from build123d import *

# Parameters (mm, degrees)
F3_W          = 55
F3_H          = 55
F4_DEPTH      = 6
F7_W          = 12.7
F7_H          = 6
F8_DEPTH      = 6
F10_W         = 12.7
F10_H         = 6
F11_DEPTH     = 6
F13_W         = 12.7
F13_H         = 6
F14_DEPTH     = 6
F16_W         = 12.7
F16_H         = 6
F17_DEPTH     = 6
F19_D         = 5
F21_D         = 5
F23_D         = 5
F25_D         = 5
F26_T4_DEPTH  = 133
F26_T10_DEPTH = 133
F26_T15_DEPTH = 133
F26_T21_DEPTH = 133
F26_T27_DEPTH = 133
F26_T33_DEPTH = 133
F26_T38_DEPTH = 133
F26_T44_DEPTH = 133
F26_T49_DEPTH = 133
F26_T55_DEPTH = 133
F26_T61_DEPTH = 133
F26_T66_DEPTH = 133
F27_R         = 6.34999


# Not quite as in the source:
# - a fillet or chamfer that OpenCascade refuses, or shapes differently, is made with other operations: its cross-section is extruded or revolved along the edge and cut away or added
# - a fillet or chamfer is up to 0.001 mm smaller than in the source, because OpenCascade refuses the exact size


with BuildPart() as f1:
    # F0 (on Front) → F1 (revolve)
    with BuildSketch(Plane.XZ):
        with BuildLine():
            Line((0, 0), (0, -32.5))
            add(Edge.make_bspline(
                [(0, -32.5), (25, -32.5), (25, 0)],
                knots=[0, 0, 0, 1.5707963268, 1.5707963268, 1.5707963268], degree=2, weights=[1, 0.7071067812, 1]))
            Line((25, 0), (0, 0))
        make_face()
        with BuildLine():
            Line((0, 0), (25, 0))
            add(Edge.make_bspline(
                [(25, 0), (25, 32.5), (0, 32.5)],
                knots=[1.5707963268, 1.5707963268, 1.5707963268, 3.1415926536, 3.1415926536, 3.1415926536], degree=2, weights=[1, 0.7071067812, 1]))
            Line((0, 32.5), (0, 0))
        make_face()
    revolve(axis=Axis((0, 0, 0), (0, 0, -1)))


with BuildPart() as f4:
    # F3 (on offset) → F4 (new body)
    with BuildSketch(Plane.XY.offset(19.05)):
        Rectangle(F3_W, F3_H)
    extrude(amount=-F4_DEPTH)

    # F5: cut F1
    add(f1.part, mode=Mode.SUBTRACT)

    # F7 (on offset) → F8 (join)
    with BuildSketch(Plane.XZ.offset(27.5)):
        with Locations((0, 16.0963926464)):
            Rectangle(F7_W, F7_H)
    extrude(amount=F8_DEPTH)

    # F10 (on offset) → F11 (join)
    with BuildSketch(Plane.YZ.offset(27.5)):
        with Locations((0, 16.087366268)):
            Rectangle(F10_W, F10_H)
    extrude(amount=F11_DEPTH)

    # F13 (on offset) → F14 (join)
    with BuildSketch(Plane.XZ.offset(-27.5)):
        with Locations((0, 16.07888937)):
            Rectangle(F13_W, F13_H)
    extrude(amount=-F14_DEPTH)

    # F16 (on offset) → F17 (join)
    with BuildSketch(Plane.YZ.offset(-27.5)):
        with Locations((0, 16.0636380315)):
            Rectangle(F16_W, F16_H)
    extrude(amount=-F17_DEPTH)

    # F19 (through all)
    with Locations(Plane.XY.offset(19.07888937)):
        with Locations((0, 28.8921689615)):
            Hole(F19_D / 2)

    # F21 (through all)
    with Locations(Plane.XY.offset(19.0636380315)):
        with Locations((-28.8809893653, 0)):
            Hole(F21_D / 2)

    # F23 (through all)
    with Locations(Plane.XY.offset(19.087366268)):
        with Locations((28.8808012381, 0)):
            Hole(F23_D / 2)

    # F25 (through all)
    with Locations(Plane.XY.offset(19.0963926464)):
        with Locations((0, -28.8607433438)):
            Hole(F25_D / 2)

    # F26: fillet of radius 25.4 on 4 edges, made by hand


with BuildPart() as f26_tool2:
    # F26_s3 → F26_t4 (new body)
    with BuildSketch(Plane.XY.offset(82.55)):
        with BuildLine():
            ThreePointArc((-27.5, 2.1), (-20.0605122421, 20.0605122421), (-2.1, 27.5))
            Line((-2.1, 27.5), (-27.5, 27.5))
            Line((-27.5, 27.5), (-27.5, 2.1))
        make_face()
    extrude(amount=-F26_T4_DEPTH)

    split(bisect_by=Plane.XZ.offset(-6.35), keep=Keep.BOTTOM)

    split(bisect_by=Plane.YZ.offset(-6.35), keep=Keep.BOTTOM)


with BuildPart() as f4_1:
    add(f4.part)

    # F26_t1: cut F26_tool2
    add(f26_tool2.part, mode=Mode.SUBTRACT)


with BuildPart() as f26_tool8:
    # F26_s9 → F26_t10 (new body)
    with BuildSketch(Plane.XY.offset(82.55)):
        with BuildLine():
            ThreePointArc((-27.5, 2.1), (-20.0605122421, 20.0605122421), (-2.1, 27.5))
            Line((-2.1, 27.5), (-27.5, 27.5))
            Line((-27.5, 27.5), (-27.5, 2.1))
        make_face()
    extrude(amount=-F26_T10_DEPTH)

    split(bisect_by=Plane.XY.offset(13.0636380315), keep=Keep.BOTTOM)


with BuildPart() as f4_2:
    add(f4_1.part)

    # F26_t7: cut F26_tool8
    add(f26_tool8.part, mode=Mode.SUBTRACT)


with BuildPart() as f26_tool13:
    # F26_s14 → F26_t15 (new body)
    with BuildSketch(Plane.XY.offset(82.55)):
        with BuildLine():
            ThreePointArc((-27.5, 2.1), (-20.0605122421, 20.0605122421), (-2.1, 27.5))
            Line((-2.1, 27.5), (-27.5, 27.5))
            Line((-27.5, 27.5), (-27.5, 2.1))
        make_face()
    extrude(amount=-F26_T15_DEPTH)

    split(bisect_by=Plane.XY.offset(13.07888937), keep=Keep.BOTTOM)

    split(bisect_by=Plane.YZ.offset(-6.35), keep=Keep.TOP)


with BuildPart() as f4_3:
    add(f4_2.part)

    # F26_t12: cut F26_tool13
    add(f26_tool13.part, mode=Mode.SUBTRACT)


with BuildPart() as f26_tool19:
    # F26_s20 → F26_t21 (new body)
    with BuildSketch(Plane.XY.offset(82.55)):
        with BuildLine():
            ThreePointArc((-2.1, -27.5), (-20.0605122421, -20.0605122421), (-27.5, -2.1))
            Line((-27.5, -2.1), (-27.5, -27.5))
            Line((-27.5, -27.5), (-2.1, -27.5))
        make_face()
    extrude(amount=-F26_T21_DEPTH)

    split(bisect_by=Plane.YZ.offset(-6.35), keep=Keep.BOTTOM)

    split(bisect_by=Plane.XZ.offset(6.35), keep=Keep.TOP)


with BuildPart() as f4_4:
    add(f4_3.part)

    # F26_t18: cut F26_tool19
    add(f26_tool19.part, mode=Mode.SUBTRACT)


with BuildPart() as f26_tool25:
    # F26_s26 → F26_t27 (new body)
    with BuildSketch(Plane.XY.offset(82.55)):
        with BuildLine():
            ThreePointArc((-2.1, -27.5), (-20.0605122421, -20.0605122421), (-27.5, -2.1))
            Line((-27.5, -2.1), (-27.5, -27.5))
            Line((-27.5, -27.5), (-2.1, -27.5))
        make_face()
    extrude(amount=-F26_T27_DEPTH)

    split(bisect_by=Plane.XY.offset(13.0963926464), keep=Keep.BOTTOM)

    split(bisect_by=Plane.XZ.offset(6.35), keep=Keep.TOP)


with BuildPart() as f4_5:
    add(f4_4.part)

    # F26_t24: cut F26_tool25
    add(f26_tool25.part, mode=Mode.SUBTRACT)


with BuildPart() as f26_tool31:
    # F26_s32 → F26_t33 (new body)
    with BuildSketch(Plane.XY.offset(82.55)):
        with BuildLine():
            ThreePointArc((-2.1, -27.5), (-20.0605122421, -20.0605122421), (-27.5, -2.1))
            Line((-27.5, -2.1), (-27.5, -27.5))
            Line((-27.5, -27.5), (-2.1, -27.5))
        make_face()
    extrude(amount=-F26_T33_DEPTH)

    split(bisect_by=Plane.XY.offset(13.0636380315), keep=Keep.BOTTOM)


with BuildPart() as f4_6:
    add(f4_5.part)

    # F26_t30: cut F26_tool31
    add(f26_tool31.part, mode=Mode.SUBTRACT)


with BuildPart() as f26_tool36:
    # F26_s37 → F26_t38 (new body)
    with BuildSketch(Plane.XY.offset(82.55)):
        with BuildLine():
            ThreePointArc((27.5, -2.1), (20.0605122421, -20.0605122421), (2.1, -27.5))
            Line((2.1, -27.5), (27.5, -27.5))
            Line((27.5, -27.5), (27.5, -2.1))
        make_face()
    extrude(amount=-F26_T38_DEPTH)

    split(bisect_by=Plane.YZ.offset(6.35), keep=Keep.TOP)

    split(bisect_by=Plane.XZ.offset(6.35), keep=Keep.TOP)


with BuildPart() as f4_7:
    add(f4_6.part)

    # F26_t35: cut F26_tool36
    add(f26_tool36.part, mode=Mode.SUBTRACT)


with BuildPart() as f26_tool42:
    # F26_s43 → F26_t44 (new body)
    with BuildSketch(Plane.XY.offset(82.55)):
        with BuildLine():
            ThreePointArc((27.5, -2.1), (20.0605122421, -20.0605122421), (2.1, -27.5))
            Line((2.1, -27.5), (27.5, -27.5))
            Line((27.5, -27.5), (27.5, -2.1))
        make_face()
    extrude(amount=-F26_T44_DEPTH)

    split(bisect_by=Plane.XY.offset(13.087366268), keep=Keep.BOTTOM)


with BuildPart() as f4_8:
    add(f4_7.part)

    # F26_t41: cut F26_tool42
    add(f26_tool42.part, mode=Mode.SUBTRACT)


with BuildPart() as f26_tool47:
    # F26_s48 → F26_t49 (new body)
    with BuildSketch(Plane.XY.offset(82.55)):
        with BuildLine():
            ThreePointArc((27.5, -2.1), (20.0605122421, -20.0605122421), (2.1, -27.5))
            Line((2.1, -27.5), (27.5, -27.5))
            Line((27.5, -27.5), (27.5, -2.1))
        make_face()
    extrude(amount=-F26_T49_DEPTH)

    split(bisect_by=Plane.XY.offset(13.0963926464), keep=Keep.BOTTOM)

    split(bisect_by=Plane.XZ.offset(6.35), keep=Keep.TOP)


with BuildPart() as f4_9:
    add(f4_8.part)

    # F26_t46: cut F26_tool47
    add(f26_tool47.part, mode=Mode.SUBTRACT)


with BuildPart() as f26_tool53:
    # F26_s54 → F26_t55 (new body)
    with BuildSketch(Plane.XY.offset(82.55)):
        with BuildLine():
            ThreePointArc((2.1, 27.5), (20.0605122421, 20.0605122421), (27.5, 2.1))
            Line((27.5, 2.1), (27.5, 27.5))
            Line((27.5, 27.5), (2.1, 27.5))
        make_face()
    extrude(amount=-F26_T55_DEPTH)

    split(bisect_by=Plane.YZ.offset(6.35), keep=Keep.TOP)

    split(bisect_by=Plane.XZ.offset(-6.35), keep=Keep.BOTTOM)


with BuildPart() as f4_10:
    add(f4_9.part)

    # F26_t52: cut F26_tool53
    add(f26_tool53.part, mode=Mode.SUBTRACT)


with BuildPart() as f26_tool59:
    # F26_s60 → F26_t61 (new body)
    with BuildSketch(Plane.XY.offset(82.55)):
        with BuildLine():
            ThreePointArc((2.1, 27.5), (20.0605122421, 20.0605122421), (27.5, 2.1))
            Line((27.5, 2.1), (27.5, 27.5))
            Line((27.5, 27.5), (2.1, 27.5))
        make_face()
    extrude(amount=-F26_T61_DEPTH)

    split(bisect_by=Plane.XY.offset(13.07888937), keep=Keep.BOTTOM)


with BuildPart() as f4_11:
    add(f4_10.part)

    # F26_t58: cut F26_tool59
    add(f26_tool59.part, mode=Mode.SUBTRACT)


with BuildPart() as f26_tool64:
    # F26_s65 → F26_t66 (new body)
    with BuildSketch(Plane.XY.offset(82.55)):
        with BuildLine():
            ThreePointArc((2.1, 27.5), (20.0605122421, 20.0605122421), (27.5, 2.1))
            Line((27.5, 2.1), (27.5, 27.5))
            Line((27.5, 27.5), (2.1, 27.5))
        make_face()
    extrude(amount=-F26_T66_DEPTH)

    split(bisect_by=Plane.XY.offset(13.087366268), keep=Keep.BOTTOM)

    split(bisect_by=Plane.XZ.offset(-6.35), keep=Keep.TOP)


with BuildPart() as f4_12:
    add(f4_11.part)

    # F26_t63: cut F26_tool64
    add(f26_tool64.part, mode=Mode.SUBTRACT)

    # F27 (radius 6.35 in the source; OpenCascade refuses exactly that, so slightly less here)
    f27_edges = [f4_12.edges().sort_by_distance(p)[0] for p in [
        (6.35, 33.5, 16.078889),
        (-6.35, 33.5, 16.078889),
        (-33.5, 6.35, 16.063638),
        (-33.5, -6.35, 16.063638),
        (-6.35, -33.5, 16.096393),
        (6.35, -33.5, 16.096393),
        (33.5, -6.35, 16.087366),
        (33.5, 6.35, 16.087366),
    ]]
    fillet(f27_edges, radius=F27_R)


solid = f4_12.part
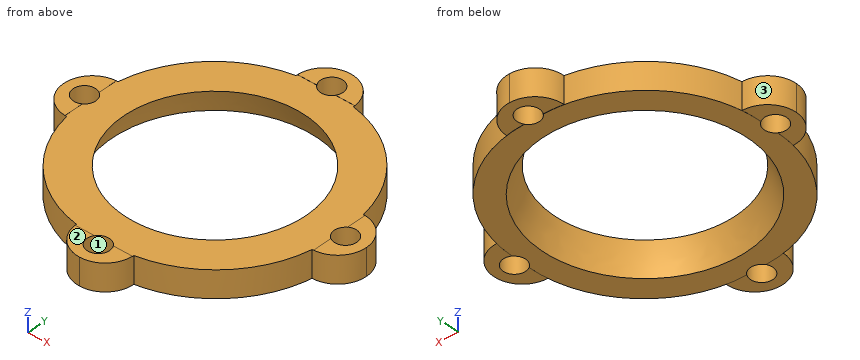
CAD build for the part. Positions are in the model's coordinates, mm. Face numbers are marked on the shaded views. Round coordinates to 2 decimals unless told otherwise and drop trailing zeros.
(1) Drop flat-ended pins along their axis: P1, Ø3, axis at y = 11.5, z = 16.5, coming from the +X side; P2, Ø3, axis at y = 23.5, z = 15, coming from the -X side; P3, Ø1, axis at y = -1, z = 18, coming from the -X side; P4, Ø3, axis at x = -28.88, y = 0, coming from the +Z side. Give the stop position or say it passes through.
(2) Slice it at A-A, the plane z = 16.5. Count the separate pieces of the cut face and the enclosed holes in it, and give its area (3 significant figures).
(3) Mould opens along X. For the marked faces 1, 2 and 3 say: pulls with the +X half, pulls with the -X half, needs draft (parallel to the pull), parting line crosses it, or undercut.
(4) Probe line 1 along X through (y, z) = (2, 14.5); line 2 along X through (y, z) = (-27.5, 16.25); line 3 along Z through (x, y) = (9.5, 21.5). List the from-to ranges inside material, lowest first.
From the geometry:
1. P1: stops at x = 26.24
1. P2: stops at x = -17.88
1. P3: stops at x = -33.48
1. P4: passes through
2. separate pieces: 1
2. enclosed holes: 5
2. area: 1,170 mm2
3. face 1: undercut
3. face 2: needs draft
3. face 3: pulls with the -X half
4. line 1: x = -33.18 to -30.38, -27.38 to -22.28, 22.28 to 27.38, 30.38 to 33.18
4. line 2: x = -6.34 to -2.1, 2.1 to 6.34
4. line 3: z = 13.05 to 19.05
